```python
from build123d import *

# Parameters (mm, degrees)
BOSS_EXTRUDE1_DEPTH = 105
BOSS_EXTRUDE2_DEPTH = 24
FILLET1_R           = 40
SKETCH5_R           = 3.219097994
BOSS_EXTRUDE3_DEPTH = 8


with BuildPart() as part:
    # Sketch1 → Boss-Extrude1 (new body)
    with BuildSketch(Plane.XY):
        Polygon((37.434072543, -12), (37.434072543, -8.558894962), (33.934072543, -12.102644962), (33.934072543, -147.897355038), (37.434072543, -151.441105038), (37.434072543, -148), (37.434072543, -147.75), (37.684072543, -147.75), (39.75, -147.75), (39.75, -12.25), (37.684072543, -12.25), (37.434072543, -12.25), align=None)
    extrude(amount=-BOSS_EXTRUDE1_DEPTH)

    # Sketch4 → Boss-Extrude2 (add)
    with BuildSketch(Plane.XY):
        Polygon((40, -152.75), (33.5, -152.75), (33.5, -7.25), (40, -7.25), (40, -80), align=None)
    extrude(amount=BOSS_EXTRUDE2_DEPTH)

    # Fillet1
    # the kernel refuses this fillet: 40 mm, written as the material it takes off along each edge
    with BuildSketch(Plane(origin=(40, 47.393732486, 24), x_dir=(0, 0, -1), z_dir=(0, -1, 0))) as fillet1_piece_1:
        with BuildLine():
            CenterArc((21.857492994, -40), FILLET1_R, 90, 33.122940208)
            Line((0, -6.5), (0, 0))
            Line((0, 0), (21.857492994, 0))
        make_face()
    extrude(amount=254.787464972, mode=Mode.SUBTRACT)

    # Sketch5 → Boss-Extrude3 (add)
    with BuildSketch(Plane(origin=(39.75, 0, 0), x_dir=(0, 0, -1), z_dir=(1, 0, 0))):
        with Locations((89.714756259, -80)):
            Circle(SKETCH5_R)
    extrude(amount=BOSS_EXTRUDE3_DEPTH)


solid = part.part
```
Work out the finished part from the listing and answer in its coordinate system (mm). A direction names the side the tool comes from. Give positions to 0.01 mm unless a question says otherwise; leave off trailing zeros. Loops run counter-clockwise (first coordinate to the right, second up) from the corner with the lowest first, then second, coordinate; pieces in that order, holes last. Notation, with made-up numbers: M -31,-5 L 9,-5 A7 cw 9,5 Z; hole C 18,16.5 d11. An arc over 180 degrees is marked long. One line per item, written item: value. Start each with the question number.
1. Find the intervals of material crossed by probe 1 along X at (y, z) = (-120, -45); probe 2 along Y at (x, z) = (39.5, -53.5); probe 3 along Y at (x, z) = (37, -59.5), in increasing order.
2. Find section A-A (y = -80). Give the vertices of the cut face in (x, z).
3. Each of these flat-tipped pins is pushed along its axis until it touches: P1, Ø2.5, axis at x = 38.5, z = -51, coming from the +Y side; P2, Ø0.7, axis at x = 38.5, z = -61, coming from the -Y side; P3, Ø1, axis at x = 41, z = -6, coming from the -Y side; P4, Ø0.6, axis at y = -74, z = 1, coming from the +X side. Where does it stop, or does it pass through?
4. Find section D-D (x = 45.5). Give the vertices of the cut face in (y, z), and give its area (3 significant figures).
5. Find section B-B (z = -4). Give the vertices of the cut face in (x, y).
6. Which of the six approach directions +Z, -Z, +X, -X, +Y, -Y give full straight-line access (tool end or side, diameter ignored) to faces 1 (the face through (35.709, -10.306, -51.765)), 2 (the face through (35.66, -149.644, -51.765)), 3 (the face through (33.934, -79, -52)), 4 (the face through (37.434, -10, -52))?
7. Find section C-C (y = -57). Give the vertices of the cut face in (x, z), and give its area (3 significant figures).
Reported:
1. probe 1: x = 33.93 to 39.75
1. probe 2: y = -147.75 to -12.25
1. probe 3: y = -151 to -9
2. outline: M 33.5,0 L 33.93,0 L 33.93,-105 L 39.75,-105 L 39.75,-92.93 L 47.75,-92.93 L 47.75,-86.5 L 39.75,-86.5 L 39.75,0 L 40,0 L 40,2.14 A40 ccw 33.5,24 Z
3. P1: stops at y = -8.56
3. P2: stops at y = -147.75
3. P3: passes through
3. P4: stops at x = 40
4. outline: C -80,-89.71 d6.44
4. area: 32.6 mm²
5. outline: M 33.93,-147.9 L 37.43,-151.44 L 37.43,-147.75 L 39.75,-147.75 L 39.75,-12.25 L 37.43,-12.25 L 37.43,-8.56 L 33.93,-12.1 Z
6. face 1: -Z, -X, +Y
6. face 2: -Z, -X, -Y
6. face 3: -Z, -X, +Y, -Y
6. face 4: -Z, +X, +Y
7. outline: M 33.5,0 L 33.93,0 L 33.93,-105 L 39.75,-105 L 39.75,0 L 40,0 L 40,2.14 A40 ccw 33.5,24 Z
7. area: 721 mm²
